Part print with two shaded views. Sizes in mm from the minimum x, y, z corner. Round coordinates to 2 decimals unless told otherwise and drop trailing zeros. One line per question, with ' | ' between items. Start each with the question number.
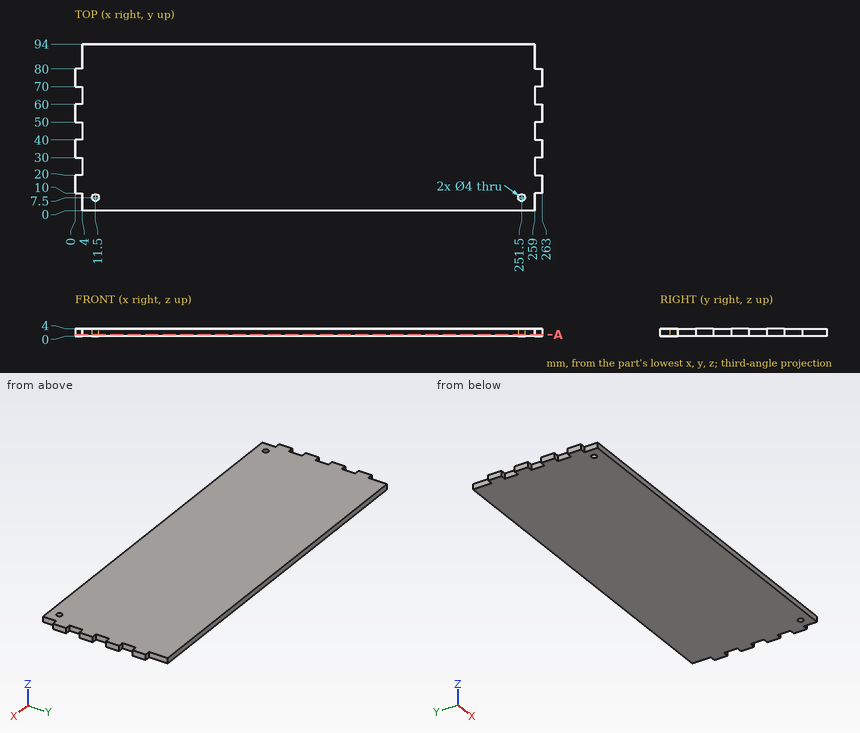
Item 1: Flat gauge pins, fed straight in: pin 1 (2.5 mm diameter, centred on x = 11.5, y = 7.5, fed in from +Z); pin 2 (2 mm diameter, centred on x = 2, z = 1.5, fed in from +Y); pin 3 (2 mm diameter, centred on y = 86.5, z = 1.5, fed in from -X); pin 4 (2 mm diameter, centred on y = 84, z = 2.5, fed in from +X). Where does each tip first touch, or does it go through?
Item 2: Wall check: line 1 along X through (y, z) = (7.5, 2.3); line 2 along Y through (x, z) = (11.5, 1.95); line 3 along X through (y, z) = (65, 0.3). Give the ranges that are in metal, low to high. Write a range as [from, to].
Item 3: Cut at A-A on z = 0.85. Count the separate pieces of the cut face and the enclosed holes in it, then the cut area to 3 significant figures.
Results found:
1) pin 1: passes through | pin 2: stops at y = 80 | pin 3: stops at x = 4 | pin 4: stops at x = 259
2) line 1: x = [4, 9.5], [13.5, 249.5], [253.5, 259] | line 2: y = [0, 5.5], [9.5, 94] | line 3: x = [4, 259]
3) separate pieces: 1 | enclosed holes: 2 | area: 24,300 mm^2
